Could you check a few things on this drawing? It's one solid part, dimensions in mm from its lowest x, y, z. A direction names the side the tool comes from. Round coordinates to 2 decimals unless told otherwise and drop trailing zeros. Write each loop counter-clockwise with the first axis right and the second up, starting at its lowest first coordinate (ties: lowest second). Pieces come first, ordered by that corner, then holes. Notation, with made-up numbers: (49, 57) -> (92, 57) arc R25 ccw to (92, 83) -> close; hole circle Ø6 at (-26.75, 80). An arc over 180 degrees is marked (long way). Put each result on its own line as item: value. Start each with the question number.
1) If I drill on line 1 along X through (y, z) = (7.75, 8); line 2 along Y through (x, z) = (7, 12.5); line 3 along Y through (x, z) = (11.25, 9.75), over which ranges is the centre line in solid material (lowest first)? Write a range as [from, to].
2) Which directions (+Z, -Z, +X, -X, +Y, -Y) give clear straight access to the entire face, cutting with the end or side of a thin tool? Please do the marked faces 1 and 2.
3) I want a section at C-C, the plane y = 15. List the corners of the cut face in (x, z) for me, then the cut area to 3 significant figures.
4) Will these pins go through, and if not, where does the flat tip stop? P1, Ø1, axis at x = 6, y = 8, coming from the -Z side; P2, Ø8, axis at y = 4, z = 12.5, coming from the -X side; P3, Ø5, axis at y = 6.5, z = 4, coming from the +X side.
5) I want a section at B-B, the plane z = 8. List the corners of the cut face in (x, y) for me.
6) I want a section at A-A, the plane x = 8. List the corners of the cut face in (y, z) for me.
7) I want a section at D-D, the plane y = 17.25. List the corners of the cut face in (x, z) for me, then the cut area to 3 significant figures.
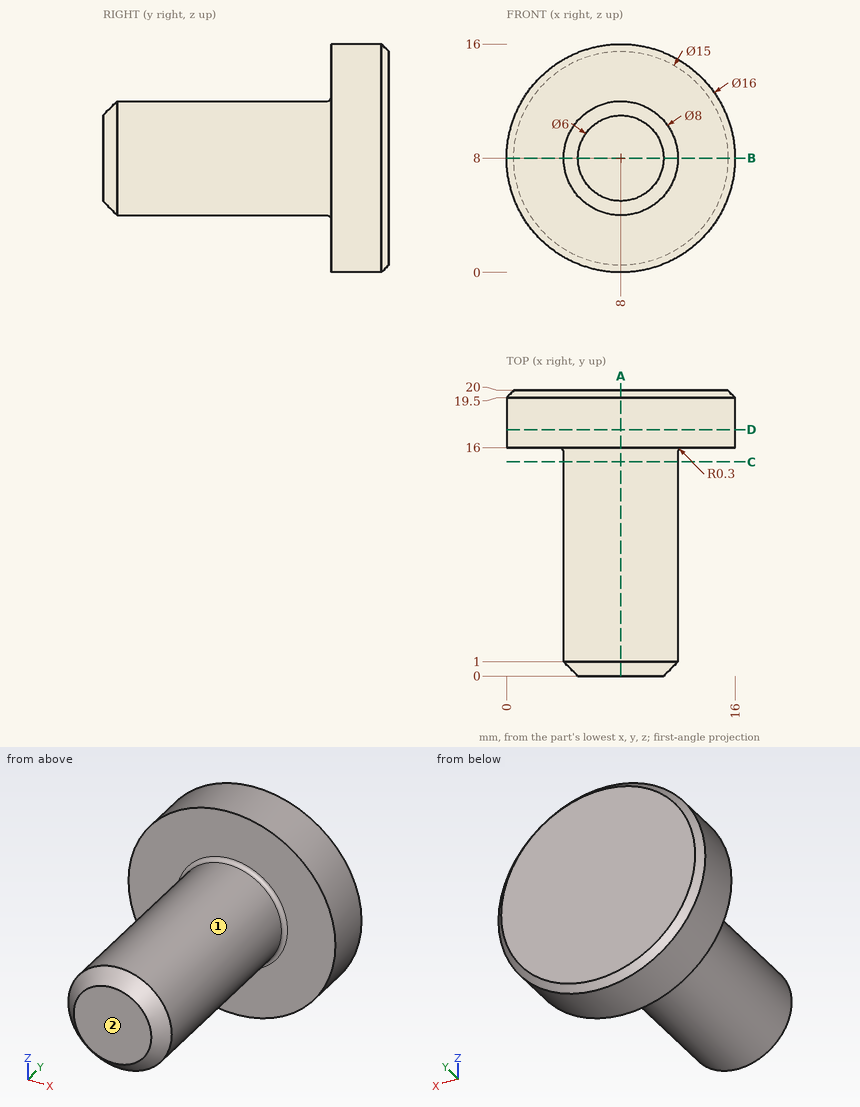
Findings:
1. line 1: x = [4, 12]
1. line 2: y = [16, 20]
1. line 3: y = [0.69, 20]
2. face 1: -Y
2. face 2: +Z, -Z, +X, -X, -Y
3. outline: circle Ø8 at (8, 8)
3. area: 50.3 mm2
4. P1: stops at z = 4.29
4. P2: stops at x = 4.03
4. P3: stops at x = 11.71
5. outline: (0, 16) -> (3.7, 16) arc R0.3 cw to (4, 15.7) -> (4, 1) -> (5, 0) -> (11, 0) -> (12, 1) -> (12, 15.7) arc R0.3 cw to (12.3, 16) -> (16, 16) -> (16, 19.5) -> (15.5, 20) -> (0.5, 20) -> (0, 19.5) -> close
6. outline: (0, 5) -> (1, 4) -> (15.7, 4) arc R0.3 cw to (16, 3.7) -> (16, 0) -> (19.5, 0) -> (20, 0.5) -> (20, 15.5) -> (19.5, 16) -> (16, 16) -> (16, 12.3) arc R0.3 cw to (15.7, 12) -> (1, 12) -> (0, 11) -> close
7. outline: circle Ø16 at (8, 8)
7. area: 201 mm2
